from build123d import *

# Parameters (mm, degrees)
BOSS_EXTRUDE1_DEPTH = 5.715


with BuildPart() as part:
    # Model → Boss-Extrude1 (new body)
    with BuildSketch(Plane.XY):
        Polygon((1288.610132665, 22.860238699), (1300.745973293, 22.860238699), (1300.745973293, 28.575245224), (1312.176695005, 28.575245224), (1312.176695005, 22.860238699), (1323.607416717, 22.860238699), (1323.607416717, 28.575245224), (1335.038138429, 28.575245224), (1335.038138429, 22.860238699), (1346.46531683, 22.860238699), (1346.46531683, 28.575245224), (1357.896038543, 28.575245224), (1357.896038543, 22.860238699), (1369.326760255, 22.860238699), (1369.326760255, 28.575245224), (1380.757481967, 28.575245224), (1380.757481967, 22.860238699), (1392.188203679, 22.860238699), (1392.188203679, 28.575245224), (1403.615382081, 28.575245224), (1403.615382081, 22.860238699), (1415.046103793, 22.860238699), (1415.046103793, 28.575245224), (1426.476825505, 28.575245224), (1426.476825505, 22.860238699), (1437.907547217, 22.860238699), (1437.907547217, 28.575245224), (1449.33826893, 28.575245224), (1449.33826893, 22.860238699), (1461.470566246, 22.860238699), (1461.470566246, 28.575245224), (1461.470566246, 51.435413056), (1461.081244935, 54.393369189), (1459.939855837, 57.150419581), (1458.123908882, 59.517571103), (1455.75520539, 61.334361366), (1453.389602295, 63.150485487), (1451.574098254, 65.517240157), (1450.429608758, 68.274290549), (1450.039844534, 71.232246682), (1450.039844534, 245.918194159), (1450.429608758, 248.876284937), (1451.574098254, 251.633200684), (1453.389602295, 254.00013252), (1455.75520539, 255.816433806), (1458.123908882, 257.633089424), (1459.939855837, 260.000375591), (1461.081244935, 262.757291337), (1461.470566246, 265.715382116), (1461.470566246, 288.575408216), (1461.470566246, 294.290414741), (1449.33826893, 294.290414741), (1449.33826893, 288.575408216), (1437.907547217, 288.575408216), (1437.907547217, 294.290414741), (1426.476825505, 294.290414741), (1426.476825505, 288.575408216), (1415.046103793, 288.575408216), (1415.046103793, 294.290414741), (1403.615382081, 294.290414741), (1403.615382081, 288.575408216), (1392.188203679, 288.575408216), (1392.188203679, 294.290414741), (1380.757481967, 294.290414741), (1380.757481967, 288.575408216), (1369.326760255, 288.575408216), (1369.326760255, 294.290414741), (1357.896038543, 294.290414741), (1357.896038543, 288.575408216), (1346.46531683, 288.575408216), (1346.46531683, 294.290414741), (1335.038138429, 294.290414741), (1335.038138429, 288.575408216), (1323.607416717, 288.575408216), (1323.607416717, 294.290414741), (1312.176695005, 294.290414741), (1312.176695005, 288.575408216), (1300.745973293, 288.575408216), (1300.745973293, 294.290414741), (1288.610132665, 294.290414741), (1288.610132665, 288.575408216), (1288.610132665, 28.575245224), align=None)
        Polygon((1444.328026989, 44.27508992), (1444.328026989, 38.560083395), (1438.612666133, 38.560083395), (1438.612666133, 49.990096445), (1444.328026989, 49.990096445), align=None, mode=Mode.SUBTRACT)
        Polygon((1444.328026989, 67.13511602), (1444.328026989, 61.420109495), (1438.612666133, 61.420109495), (1438.612666133, 72.850122545), (1444.328026989, 72.850122545), align=None, mode=Mode.SUBTRACT)
        Polygon((1444.328026989, 89.99514212), (1444.328026989, 84.280135595), (1438.612666133, 84.280135595), (1438.612666133, 95.710148645), (1444.328026989, 95.710148645), align=None, mode=Mode.SUBTRACT)
        Polygon((1444.328026989, 112.85516822), (1444.328026989, 107.140161695), (1438.612666133, 107.140161695), (1438.612666133, 118.570174745), (1444.328026989, 118.570174745), align=None, mode=Mode.SUBTRACT)
        Polygon((1444.328026989, 135.71519432), (1444.328026989, 130.000187795), (1438.612666133, 130.000187795), (1438.612666133, 141.430200846), (1444.328026989, 141.430200846), align=None, mode=Mode.SUBTRACT)
        Polygon((1444.328026989, 158.575220421), (1444.328026989, 152.860213896), (1438.612666133, 152.860213896), (1438.612666133, 164.290226946), (1444.328026989, 164.290226946), align=None, mode=Mode.SUBTRACT)
        Polygon((1444.328026989, 181.435246521), (1444.328026989, 175.720239996), (1438.612666133, 175.720239996), (1438.612666133, 187.150253046), (1444.328026989, 187.150253046), align=None, mode=Mode.SUBTRACT)
        Polygon((1444.328026989, 204.295272621), (1444.328026989, 198.580266096), (1438.612666133, 198.580266096), (1438.612666133, 210.010279146), (1444.328026989, 210.010279146), align=None, mode=Mode.SUBTRACT)
        Polygon((1444.328026989, 227.155298721), (1444.328026989, 221.440292196), (1438.612666133, 221.440292196), (1438.612666133, 232.870305246), (1444.328026989, 232.870305246), align=None, mode=Mode.SUBTRACT)
        Polygon((1444.328026989, 250.015324821), (1444.328026989, 244.300318296), (1438.612666133, 244.300318296), (1438.612666133, 255.730331346), (1444.328026989, 255.730331346), align=None, mode=Mode.SUBTRACT)
        Polygon((1444.328026989, 272.875350921), (1444.328026989, 267.160344396), (1438.612666133, 267.160344396), (1438.612666133, 278.590357446), (1444.328026989, 278.590357446), align=None, mode=Mode.SUBTRACT)
    extrude(amount=BOSS_EXTRUDE1_DEPTH)


solid = part.part
Input: part model. Units: mm. Frame: model coordinates. A direction names the side the tool comes from. Give positions to 0.01 mm unless a question says otherwise; leave off trailing zeros. Order: outer loops, then holes, each group sorted by start corner. A loop starts at its lowest first (then second) coordinate and runs counter-clockwise, first axis right, second up. Notation, with made-up numbers: (64.5, 78.25) -> (78.5, 78.25) arc R19 cw to (78.5, 114.25) -> close; hole circle Ø9 at (8, -38). An arc over 180 degrees is marked (long way). Use one line per item in the form item = value.
1) Mould query, pull axis X, two halves, no side actions, for faces 1 (the flat face through (1288.61, 160, 3)), 2 (the flat face through (1352, 288.575, 3)), 3 (the flat face through (1409, 294.29, 3)). Classes: pulls with the +X half, pulls with the -X half, needs draft (parallel to the pull), parting line crosses it, or undercut.
Response values:
face_1 = pulls with the -X half
face_2 = undercut
face_3 = needs draft
2) Section A-A, the plane y = 276. Return loops of the section in (x, z) (3 decimals).
Response values:
outline = (1288.61, 0) -> (1438.613, 0) -> (1438.613, 5.715) -> (1288.61, 5.715) -> close; (1444.328, 0) -> (1461.471, 0) -> (1461.471, 5.715) -> (1444.328, 5.715) -> close
3) Line query: probe 1 along X at (y, z) = (87, 5.15); probe 2 along Y at (x, z) = (1327.5, 4.75); probe 3 along X at (y, z) = (212.5, 4.95). Output: solid intervals per line, ascending.
Response values:
probe_1 = 1288.61 to 1438.61, 1444.33 to 1450.04
probe_2 = 28.58 to 288.58
probe_3 = 1288.61 to 1450.04
4) First-contact query: pin 1 Ø2 at (x, z) = (1422, 3.5) entering from -Y; pin 2 Ø1.7 at (x, z) = (1441.5, 2) entering from +Y; pin 3 Ø1 at (y, z) = (212.5, 4) entering from +X. Flat tips, straight axial feed; report the tip coordinate or a pass-through.
Response values:
pin_1 = 28.58
pin_2 = 288.58
pin_3 = 1450.04
5) Section B-B, the plane y = 228. Return loops of the section in (x, z) (3 decimals).
Response values:
outline = (1288.61, 0) -> (1438.613, 0) -> (1438.613, 5.715) -> (1288.61, 5.715) -> close; (1444.328, 0) -> (1450.04, 0) -> (1450.04, 5.715) -> (1444.328, 5.715) -> close
6) Section C-C, the plane z = 2.15. Count the separate pieces of the cut face and the enclosed holes in it, and give its area (3 significant figures).
Response values:
separate_pieces = 1
enclosed_holes = 11
area = 43,100 mm^2
7) Reachability of faces 4 (the flat face through (1364, 294.29, 3)), 5 (the flat face through (1318, 22.86, 3)), 6 (the flat face through (1437.908, 291, 3)), 7 (the flat face through (1415.046, 26, 3)), 8 (the flat face through (1442, 152.86, 3)) from +Z, -Z, +X, -X, +Y, -Y: full face, straight path, thin tool, end or side. Return the list, or none.
Response values:
face_4 = +Z, -Z, +X, -X, +Y
face_5 = +Z, -Z, +X, -X, -Y
face_6 = +Z, -Z, +Y
face_7 = +Z, -Z, -Y
face_8 = +Z, -Z
8) Section D-D, the plane y = 170.5. Return loops of the section in (x, z) (3 decimals), and give its area (3 significant figures).
Response values:
outline = (1288.61, 0) -> (1450.04, 0) -> (1450.04, 5.715) -> (1288.61, 5.715) -> close
area = 923 mm^2
